Geometry: final body of the model. Coordinates: model frame, mm. Face numbers are marked on the shaded views. A direction names the side the tool comes from. Give positions to 0.01 mm unless a question says otherwise; leave off trailing zeros. Write each loop counter-clockwise with the first axis right and the second up, starting at its lowest first coordinate (ties: lowest second). Pieces come first, ordered by that corner, then holes. Notation, with made-up numbers: (12.25, -30.5) -> (47.25, -30.5) arc R22 cw to (47.25, -0.5) -> close; hole circle Ø11 at (-14.75, 16). An arc over 180 degrees is marked (long way). Answer as a JSON object with one key per item and string values.
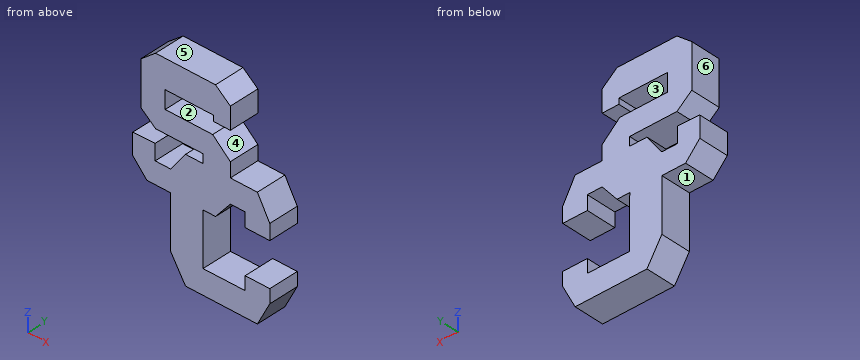
from build123d import *

# Parameters (mm, degrees)
F1_DEPTH = 25


with BuildPart() as f1:
    # F0 (on Front) → F1 (new body)
    with BuildSketch(Plane.XZ):
        Polygon((25, 54.390011), (-25, 54.390011), (-37.401415, 44.280367), (-37.401415, 7.760552), (-25, -2.349091), (14.553074, -2.349091), (14.553074, -9.739744), (37.401415, -9.739744), (37.401415, 2.495785), (22.646608, 15.901208), (-16.990989, 15.901208), (-16.990989, 30.78134), (23.416273, 30.78134), (23.416273, 26.035091), (37.401415, 26.035091), (37.401415, 44.280367), align=None)
        Polygon((37.401415, -9.739744), (14.553074, -9.739744), (14.553074, -26.700841), (-12.420272, -26.700841), (-25.357073, -26.700841), (-25.357073, -13.520215), (-44.085521, -14.033324), (-44.085521, -31.581496), (-32.246049, -44.583419), (-12.420272, -44.583419), (14.358093, -44.583419), (25, -44.583419), (37.401415, -29.370707), align=None)
        Polygon((14.553074, -26.700841), (14.553074, -9.739744), (0, -9.739744), (-12.420272, -26.700841), align=None)
        Polygon((59.962764, -9.739744), (37.401415, -9.739744), (37.401415, -29.370707), (49.803725, -29.370707), (49.803725, -41.213728), (70.303194, -41.213728), (70.303194, -28.267196), align=None)
        Polygon((14.553074, -88.711776), (14.358093, -44.583419), (-12.420272, -44.583419), (-12.420272, -88.711776), (0, -108.790196), (59.962764, -108.790196), (70.303194, -88.711776), (70.303194, -77.314541), (49.803725, -77.314541), (49.803725, -88.556021), align=None)
    extrude(amount=F1_DEPTH)


solid = f1.part
Q1. Cut plane C-C (x = 46.5). Return the cut outline in (y, z), and give its area (3 significant figures).
Values:
{"outline": "(-25, -108.79) -> (0, -108.79) -> (0, -88.57) -> (-25, -88.57) -> close; (-25, -29.37) -> (0, -29.37) -> (0, -9.74) -> (-25, -9.74) -> close", "area": "996 mm²"}
Q2. Set-up query: the marked faces 1, 2 and 3. Return all of +Z, -Z, +X, -X, +Y, -Y with unobstructed straight access to the full face (end or side cutting, diameter ignored); none if empty.
Values:
{"face 1": "-Z, -X, +Y, -Y", "face 2": "+X, +Y, -Y", "face 3": "+Y, -Y"}
Q3. Cut plane B-B (z = -36). Return the cut outline in (x, y).
Values:
{"outline": "(-40.06, -25) -> (32, -25) -> (32, 0) -> (-40.06, 0) -> close; (49.8, -25) -> (70.3, -25) -> (70.3, 0) -> (49.8, 0) -> close"}
Q4. Cut plane A-A (x = 8). Return the cut outline in (y, z), and give its area (3 significant figures).
Values:
{"outline": "(-25, -108.79) -> (0, -108.79) -> (0, -9.74) -> (-25, -9.74) -> close; (-25, -2.35) -> (0, -2.35) -> (0, 15.9) -> (-25, 15.9) -> close; (-25, 30.78) -> (0, 30.78) -> (0, 54.39) -> (-25, 54.39) -> close", "area": "3,520 mm²"}
Q5. Cut plane D-D (z = 40). Return the cut outline in (x, y), and give its area (3 significant figures).
Values:
{"outline": "(-37.4, -25) -> (37.4, -25) -> (37.4, 0) -> (-37.4, 0) -> close", "area": "1,870 mm²"}
Q6. Mould query, pull axis Z, two halves, no side actions, for the marked faces 4, 5 and 6. Classes: pulls with the +Z half, pulls with the -Z half, needs draft (parallel to the pull), parting line crosses it, or undercut.
Values:
{"face 4": "undercut", "face 5": "pulls with the +Z half", "face 6": "needs draft"}
Q7. Material intervals for L1, parallel to Z at x = 5, y = -21.5; L2, parallel to Z at x = -13, y = -16; L3, parallel to Z at x = -20, y = -5.25, sorted ascending. Write a range as from..to.
Values:
{"L1": "-108.79..-9.74, -2.35..15.9, 30.78..54.39", "L2": "-44.58..-26.7, -2.35..15.9, 30.78..54.39", "L3": "-44.58..-26.7, -2.35..54.39"}
Q8. First-contact query: P1, Ø1.5, axis at y = -7.5, z = 32, coming from the -X side; P2, Ø12.5, axis at y = -17.5, z = -84, coming from the -X side; P3, Ø1, axis at x = -32, y = -18.5, coming from the -Z side; P4, Ø6, axis at y = -12.5, z = -32.5, coming from the -X side. Flat tips, straight axial feed; report the tip coordinate or a pass-through.
Values:
{"P1": "x = -37.4", "P2": "x = -12.42", "P3": "z = -44.58", "P4": "x = -44.09"}
